Could you check a few things on this model? Use its own coordinates, in mm. Face numbers are marked on the shaded views. Give positions to 0.01 mm unless a question says otherwise; leave off trailing zeros. Loops run counter-clockwise (first coordinate to the right, second up) from the corner with the lowest first, then second, coordinate; pieces in that order, holes last. Notation, with made-up numbers: (20.5, -23) -> (44.5, -23) arc R32 ccw to (44.5, 14) -> close; hole circle Ø8 at (33, 7). An arc over 180 degrees is marked (long way). Put each result on its own line as item: value.
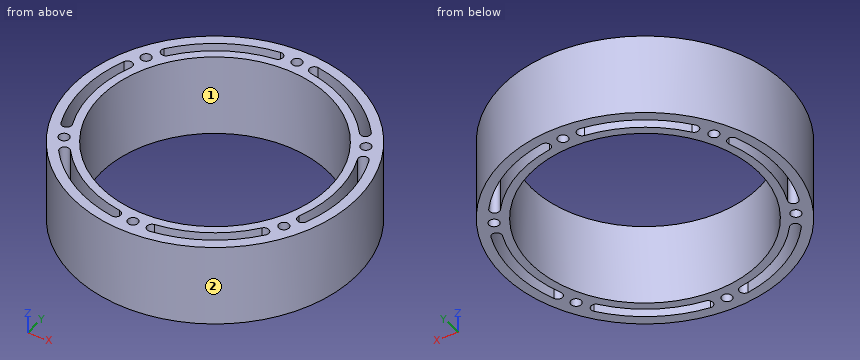
```python
from build123d import *

# Parameters (mm, degrees)
HOLE_START                        = -12.5
HOLE_WIZARD_3_1_3_1_6_OUTLINE_R   = 43
HOLE_WIZARD_3_1_3_1_6_OUTLINE_R_2 = 1.55
HOLE_WIZARD_3_1_3_1_6_DEPTH       = 25
HOLE_WIZARD_3_1_3_1_5_D           = 3.1
HOLE_WIZARD_3_1_3_1_4_D           = 3.1
HOLE_WIZARD_3_1_3_1_3_D           = 3.1
HOLE_WIZARD_3_1_3_1_2_D           = 3.1
HOLE_WIZARD_3_1_3_1_1_D           = 3.1
HOLE_WIZARD_M64_1_D               = 69


with BuildPart() as part:
    # Ø3.1 (3.1) 直径孔6: read off the stored shape, not the designer's step
    # Ø3.1 (3.1) 直径孔6 outline → Ø3.1 (3.1) 直径孔6 (new body)
    with BuildSketch(Plane.XY.offset(HOLE_START)):
        Circle(HOLE_WIZARD_3_1_3_1_6_OUTLINE_R)
        with BuildLine():
            ThreePointArc((-31.420080332, -24.7543643), (-31.170115981, -22.647822626), (-29.063574308, -22.897786978))
            ThreePointArc((-29.063574308, -22.897786978), (-18.5, -32.04293994), (-5.298278059, -36.618687164))
            ThreePointArc((-5.298278059, -36.618687164), (-4.028531744, -38.318023592), (-5.727868172, -39.587769907))
            ThreePointArc((-5.727868172, -39.587769907), (-20, -34.641016151), (-31.420080332, -24.7543643))
        make_face(mode=Mode.SUBTRACT)
        with Locations((0, -38.5)):
            Circle(HOLE_WIZARD_3_1_3_1_6_OUTLINE_R_2, mode=Mode.SUBTRACT)
        with BuildLine():
            ThreePointArc((5.727868172, -39.587769907), (4.028531744, -38.318023592), (5.298278059, -36.618687164))
            ThreePointArc((5.298278059, -36.618687164), (18.5, -32.04293994), (29.063574308, -22.897786978))
            ThreePointArc((29.063574308, -22.897786978), (31.170115981, -22.647822626), (31.420080332, -24.7543643))
            ThreePointArc((31.420080332, -24.7543643), (20, -34.641016151), (5.727868172, -39.587769907))
        make_face(mode=Mode.SUBTRACT)
        with BuildLine():
            ThreePointArc((-37.147948505, 14.833405607), (-35.198647726, 15.670200965), (-34.361852367, 13.720900186))
            ThreePointArc((-34.361852367, 13.720900186), (-37, 0), (-34.361852367, -13.720900186))
            ThreePointArc((-34.361852367, -13.720900186), (-35.198647726, -15.670200965), (-37.147948505, -14.833405607))
            ThreePointArc((-37.147948505, -14.833405607), (-40, 0), (-37.147948505, 14.833405607))
        make_face(mode=Mode.SUBTRACT)
        with BuildLine():
            ThreePointArc((-5.727868172, 39.587769907), (-4.028531744, 38.318023592), (-5.298278059, 36.618687164))
            ThreePointArc((-5.298278059, 36.618687164), (-18.5, 32.04293994), (-29.063574308, 22.897786978))
            ThreePointArc((-29.063574308, 22.897786978), (-31.170115981, 22.647822626), (-31.420080332, 24.7543643))
            ThreePointArc((-31.420080332, 24.7543643), (-20, 34.641016151), (-5.727868172, 39.587769907))
        make_face(mode=Mode.SUBTRACT)
        with BuildLine():
            ThreePointArc((37.147948505, -14.833405607), (35.198647726, -15.670200965), (34.361852367, -13.720900186))
            ThreePointArc((34.361852367, -13.720900186), (37, 0), (34.361852367, 13.720900186))
            ThreePointArc((34.361852367, 13.720900186), (35.198647726, 15.670200965), (37.147948505, 14.833405607))
            ThreePointArc((37.147948505, 14.833405607), (40, 0), (37.147948505, -14.833405607))
        make_face(mode=Mode.SUBTRACT)
        with BuildLine():
            ThreePointArc((31.420080332, 24.7543643), (31.170115981, 22.647822626), (29.063574308, 22.897786978))
            ThreePointArc((29.063574308, 22.897786978), (18.5, 32.04293994), (5.298278059, 36.618687164))
            ThreePointArc((5.298278059, 36.618687164), (4.028531744, 38.318023592), (5.727868172, 39.587769907))
            ThreePointArc((5.727868172, 39.587769907), (20, 34.641016151), (31.420080332, 24.7543643))
        make_face(mode=Mode.SUBTRACT)
    extrude(amount=HOLE_WIZARD_3_1_3_1_6_DEPTH)

    # Ø3.1 (3.1) 直径孔5 (through all)
    with Locations(Plane.XY.offset(12.5)):
        with Locations((33.341978046, -19.25)):
            Hole(HOLE_WIZARD_3_1_3_1_5_D / 2)

    # Ø3.1 (3.1) 直径孔4 (through all)
    with Locations(Plane.XY.offset(12.5)):
        with Locations((33.341978046, 19.25)):
            Hole(HOLE_WIZARD_3_1_3_1_4_D / 2)

    # Ø3.1 (3.1) 直径孔3 (through all)
    with Locations(Plane.XY.offset(12.5)):
        with Locations((0, 38.5)):
            Hole(HOLE_WIZARD_3_1_3_1_3_D / 2)

    # Ø3.1 (3.1) 直径孔2 (through all)
    with Locations(Plane.XY.offset(12.5)):
        with Locations((-33.341978046, 19.25)):
            Hole(HOLE_WIZARD_3_1_3_1_2_D / 2)

    # Ø3.1 (3.1) 直径孔1 (through all)
    with Locations(Plane.XY.offset(12.5)):
        with Locations((-33.341978046, -19.25)):
            Hole(HOLE_WIZARD_3_1_3_1_1_D / 2)

    # M64 间隙孔1 (through all)
    with Locations(Plane(origin=(0, 0, -12.5), x_dir=(-1, 0, 0), z_dir=(0, 0, -1))):
        with Locations((0, 0)):
            Hole(HOLE_WIZARD_M64_1_D / 2)


solid = part.part
```
1. If we section it at B-B (x = 0): List the corners of the cut face in (y, z) for me.
Recorded:
outline: (-43, -12.5) -> (-40.05, -12.5) -> (-40.05, 12.5) -> (-43, 12.5) -> close; (-36.95, -12.5) -> (-34.5, -12.5) -> (-34.5, 12.5) -> (-36.95, 12.5) -> close; (34.5, -12.5) -> (36.95, -12.5) -> (36.95, 12.5) -> (34.5, 12.5) -> close; (40.05, -12.5) -> (43, -12.5) -> (43, 12.5) -> (40.05, 12.5) -> close
2. Thinking about a two-plate mould opening in Y: for the marked faces 1 and 2, which applies, pulls with the +Y half, pulls with the -Y half, needs draft (parallel to the pull), parting line crosses it, or undercut?
Recorded:
face 1: undercut
face 2: parting line crosses it
3. I'm going to push flat-ended pins straight in: pin 1 (6 mm diameter, centred on y = 11.5, z = 7, fed in from +X); pin 2 (3.5 mm diameter, centred on x = -33.34, y = 19.25, fed in from -Z); pin 3 (1.5 mm diameter, centred on x = 10, z = 7.5, fed in from -Y); pin 4 (10 mm diameter, centred on y = -31, z = -2, fed in from -X). Where does each tip first touch, or does it pass through?
Recorded:
pin 1: stops at x = 42.15
pin 2: stops at z = -12.5
pin 3: stops at y = -41.99
pin 4: stops at x = -34.25
4. If we section it at C-C (y = -19.25): List the corners of the cut face in (x, z) for me.
Recorded:
outline: (-38.45, -12.5) -> (-34.89, -12.5) -> (-34.89, 12.5) -> (-38.45, 12.5) -> close; (-31.79, -12.5) -> (-28.63, -12.5) -> (-28.63, 12.5) -> (-31.79, 12.5) -> close; (28.63, -12.5) -> (31.79, -12.5) -> (31.79, 12.5) -> (28.63, 12.5) -> close; (34.89, -12.5) -> (38.45, -12.5) -> (38.45, 12.5) -> (34.89, 12.5) -> close
5. If we section it at A-A (z = -9.5): Count the separate pieces of the cut face and the enclosed holes in it, then the cut area to 3 significant figures.
Recorded:
separate pieces: 1
enclosed holes: 13
area: 1,460 mm^2
6. I need wall thicknesses on line 1 (X direction, y = 25.5, z = -9); line 2 (Y direction, x = -21, z = -10.5); line 3 (X direction, y = 14.5, z = 4.5). Which ranges of each line are inside material? Lowest first, please.
Recorded:
line 1: x = -34.62 to -30.82, -26.81 to -23.24, 23.24 to 26.81, 30.82 to 34.62
line 2: y = -37.52 to -34.04, -30.46 to -27.37, 27.37 to 30.46, 34.04 to 37.52
line 3: x = -40.48 to -37.28, -34.27 to -31.3, 31.3 to 34.27, 37.28 to 40.48
